```python
from build123d import *

# Parameters (mm, degrees)
SKETCH_1_R          = 10
EXTRUDE_1_DEPTH     = 3
SKETCH_2_R          = 5
EXTRUDE_2_DEPTH     = 2
SKETCH_3_R          = 1.6
SKETCH_3_R_2        = 1
CUT_EXTRUDE_1_DEPTH = 6
SKETCH_4_R          = 3
CUT_EXTRUDE_2_DEPTH = 3


with BuildPart() as part:
    # 草图1 → 凸台-拉伸1 (new body)
    with BuildSketch(Plane(origin=(0, 0, 0), x_dir=(1, 0, 0), z_dir=(0, 1, 0))):
        Circle(SKETCH_1_R)
    extrude(amount=EXTRUDE_1_DEPTH)

    # 草图2 → 凸台-拉伸2 (add)
    with BuildSketch(Plane(origin=(0, 3, 0), x_dir=(1, 0, 0), z_dir=(0, 1, 0))):
        Circle(SKETCH_2_R)
    extrude(amount=EXTRUDE_2_DEPTH)

    # 草图3 → 切除-拉伸1 (cut, through all)
    with BuildSketch(Plane.XZ):
        Circle(SKETCH_3_R)
        with Locations((0, 8)):
            Circle(SKETCH_3_R_2)
        with Locations((5.656854249, 5.656854249)):
            Circle(SKETCH_3_R_2)
        with Locations((8, 0)):
            Circle(SKETCH_3_R_2)
        with Locations((5.656854249, -5.656854249)):
            Circle(SKETCH_3_R_2)
        with Locations((0, -8)):
            Circle(SKETCH_3_R_2)
        with Locations((-5.656854249, -5.656854249)):
            Circle(SKETCH_3_R_2)
        with Locations((-8, 0)):
            Circle(SKETCH_3_R_2)
        with Locations((-5.656854249, 5.656854249)):
            Circle(SKETCH_3_R_2)
    extrude(amount=-CUT_EXTRUDE_1_DEPTH, mode=Mode.SUBTRACT)

    # 草图4 → 切除-拉伸2 (cut)
    with BuildSketch(Plane.XZ):
        Circle(SKETCH_4_R)
    extrude(amount=-CUT_EXTRUDE_2_DEPTH, mode=Mode.SUBTRACT)


solid = part.part
```
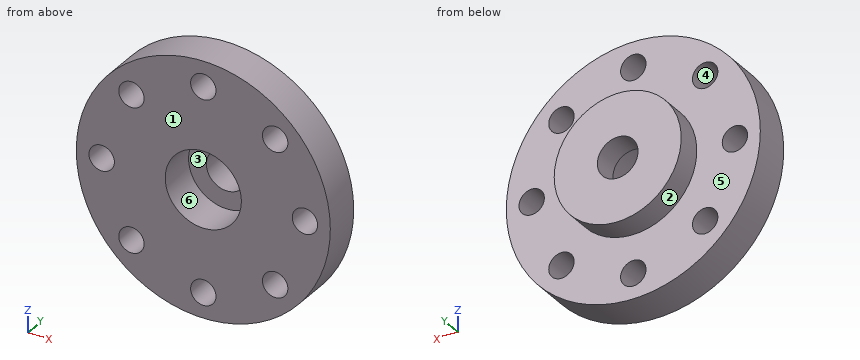
Geometry check sheet. Reference: the model listing, model coordinates, mm. Face numbers are marked on the shaded views. A direction names the side the tool comes from. Round coordinates to 2 decimals unless told otherwise and drop trailing zeros. Loops run counter-clockwise (first coordinate to the right, second up) from the corner with the lowest first, then second, coordinate; pieces in that order, holes last. Notation, with made-up numbers: (-20.75, -21) - (29.25, -21) arc R15 ccw to (29.25, -7) - close; hole circle Ø6 at (70.25, 62.5). An arc over 180 degrees is marked (long way). Write item = value, one per line. Start each with the question number.
1. Section check A-A on x = 0. Enter the section's corners in (y, z).
2. Mould release check, pull along X, two halves, no side actions. Record for the marked faces 1, 2 and 3: released by +X, released by -X, zero draft, split by the parting line, or undercut.
3. Section check D-D on y = 1.3. Give the number of separate pieces and of enclosed holes in the cut face, then the cut area to 3 significant figures.
4. Set-up check for the marked faces 4, 5 and 6: record each of +Z, -Z, +X, -X, +Y, -Y from which the full face is reachable in a straight line by a thin tool's end or side.
5. Depth check by flat-ended pin: pin 1 (3 mm diameter, centred on x = 0, z = 8, fed in from +Y); pin 2 (3 mm diameter, centred on x = 4.5, y = 2.5, fed in from +Z); pin 3 (1.9 mm diameter, centred on x = 0, z = 0, fed in from -Y); pin 4 (2 mm diameter, centred on x = -8, y = 2.5, fed in from -Z). Enter the tip coordinate at first touch or a pass-through.
6. Thickness scan on line 1 (Z direction, x = 0, y = 1); line 2 (Z direction, x = -0.75, y = 1.8); line 3 (X direction, y = 1.3, z = -5.75). Record the ranges inside material, lowest first.
7. Section check B-B on x = 8. Enter the section's corners in (y, z), then the cut area to 3 significant figures.
8. Section check C-C on z = 8. Enter the section's corners in (x, y).
Working result:
q1.outline = (0, -10) - (3, -10) - (3, -9) - (0, -9) - close; (0, -7) - (3, -7) - (3, -5) - (5, -5) - (5, -1.6) - (3, -1.6) - (3, -3) - (0, -3) - close; (0, 3) - (3, 3) - (3, 1.6) - (5, 1.6) - (5, 5) - (3, 5) - (3, 7) - (0, 7) - close; (0, 9) - (3, 9) - (3, 10) - (0, 10) - close
q2.face_1 = zero draft
q2.face_2 = split by the parting line
q2.face_3 = undercut
q3.separate_pieces = 1
q3.enclosed_holes = 9
q3.area = 261 mm^2
q4.face_4 = +Y, -Y
q4.face_5 = +Y
q4.face_6 = -Y
q5.pin_1 = 3
q5.pin_2 = 9.54
q5.pin_3 = through
q5.pin_4 = -7.14
q6.line_1 = -10 to -9, -7 to -3, 3 to 7, 9 to 10
q6.line_2 = -9.97 to -8.66, -7.34 to -2.9, 2.9 to 7.34, 8.66 to 9.97
q6.line_3 = -8.18 to -6.65, -4.66 to 4.66, 6.65 to 8.18
q7.outline = (0, -6) - (3, -6) - (3, -1) - (0, -1) - close; (0, 1) - (3, 1) - (3, 6) - (0, 6) - close
q7.area = 30.0 mm^2
q8.outline = (-6, 0) - (-1, 0) - (-1, 3) - (-6, 3) - close; (1, 0) - (6, 0) - (6, 3) - (1, 3) - close
